```python
from build123d import *

# Parameters (mm, degrees)
SKETCH1_W           = 90
SKETCH1_H           = 60
SKETCH1_W_2         = 13.5
SKETCH1_H_2         = 54
SKETCH1_W_3         = 59.25
SKETCH1_H_3         = 43
BOSS_EXTRUDE3_DEPTH = 1.25
SKETCH1_6_W         = 100
SKETCH1_6_H         = 70
SKETCH1_6_R         = 1.5
SKETCH1_6_W_2       = 90
SKETCH1_6_H_2       = 60
BOSS_EXTRUDE4_DEPTH = 2.5


with BuildPart() as part:
    # Sketch1 → Boss-Extrude3 (new body)
    with BuildSketch(Plane.XY):
        with Locations((45, 30)):
            Rectangle(SKETCH1_W, SKETCH1_H)
        with Locations((81.5, 30.5)):
            Rectangle(SKETCH1_W_2, SKETCH1_H_2, mode=Mode.SUBTRACT)
        with Locations((38.125, 30)):
            Rectangle(SKETCH1_W_3, SKETCH1_H_3, mode=Mode.SUBTRACT)
    extrude(amount=-BOSS_EXTRUDE3_DEPTH)

    # Sketch1_6 → Boss-Extrude4 (add)
    with BuildSketch(Plane.XY):
        with Locations((45, 30)):
            Rectangle(SKETCH1_6_W, SKETCH1_6_H)
        with Locations((92.5, -2.5)):
            Circle(SKETCH1_6_R, mode=Mode.SUBTRACT)
        with Locations((92.5, 62.5)):
            Circle(SKETCH1_6_R, mode=Mode.SUBTRACT)
        with Locations((-2.5, 62.5)):
            Circle(SKETCH1_6_R, mode=Mode.SUBTRACT)
        with Locations((-2.5, -2.5)):
            Circle(SKETCH1_6_R, mode=Mode.SUBTRACT)
        with Locations((45, 30)):
            Rectangle(SKETCH1_6_W_2, SKETCH1_6_H_2, mode=Mode.SUBTRACT)
    extrude(amount=-BOSS_EXTRUDE4_DEPTH)


solid = part.part
```
Could you check a few things on this model? Use its own coordinates, in mm. A direction names the side the tool comes from. Coordinates: 2 decimals unless noted, no trailing zeros. Order: outer loops, then holes, each group sorted by start corner. A loop starts at its lowest first (then second) coordinate and runs counter-clockwise, first axis right, second up. Notation, with made-up numbers: M 78,-40 L 132,-40 A10 cw 132,-26 Z; hole C 77.5,5.25 d2. An arc over 180 degrees is marked long. Use a Markdown table: item, result. Add a question column.
Q1. Which directions (+Z, -Z, +X, -X, +Y, -Y) give clear straight access to the entire face, cutting with the end or side of a thin tool? Please do faces 4 (the flat face through (34, 4, -1.25)), 5 (the cylindrical face through (93.306, 63.765, -1.232)).
Q2. I want a section at D-D on y = 62.5. List the corners of the cut face in (x, z) for me, then the cut area to 3 significant figures.
Q3. I want a section at C-C on x = -2.5. List the corners of the cut face in (y, z) for me.
Q4. If I drill on L1, parallel to Y at x = 92.5, z = -1.55; L2, parallel to X at y = 40.5, z = -0.8; L3, parallel to X at y = 51, z = -1.8, over which ranges is the centre line in solid material (lowest first)?
Q5. I want a section at A-A on x = 84. List the corners of the cut face in (y, z) for me.
Q6. I want a section at B-B on y = 16. List the corners of the cut face in (x, z) for me.
Q7. We'd pull the mould along Y, two halves only. Please class faces 1 (the flat face through (44, 54, 0)), 2 (the flat face through (44, 65, -1)), 3 (the cylindrical face through (-2.695, 63.987, -1.232)): pulls with the +Y half, pulls with the -Y half, needs draft (parallel to the pull), parting line crosses it, or undercut.
Checked values:
| question | item | result |
|---|---|---|
| 1 | face 4 | -Z |
| 1 | face 5 | +Z, -Z |
| 2 | outline | M -5,-2.5 L -4,-2.5 L -4,0 L -5,0 Z; M -1,-2.5 L 91,-2.5 L 91,0 L -1,0 Z; M 94,-2.5 L 95,-2.5 L 95,0 L 94,0 Z |
| 2 | area | 235 mm² |
| 3 | outline | M -5,-2.5 L -4,-2.5 L -4,0 L -5,0 Z; M -1,-2.5 L 61,-2.5 L 61,0 L -1,0 Z; M 64,-2.5 L 65,-2.5 L 65,0 L 64,0 Z |
| 4 | L1 | -5 to -4, -1 to 61, 64 to 65 |
| 4 | L2 | -5 to 8.5, 67.75 to 74.75, 88.25 to 95 |
| 4 | L3 | -5 to 0, 90 to 95 |
| 5 | outline | M -5,-2.5 L 0,-2.5 L 0,-1.25 L 3.5,-1.25 L 3.5,0 L -5,0 Z; M 57.5,-1.25 L 60,-1.25 L 60,-2.5 L 65,-2.5 L 65,0 L 57.5,0 Z |
| 6 | outline | M -5,-2.5 L 0,-2.5 L 0,-1.25 L 8.5,-1.25 L 8.5,0 L -5,0 Z; M 67.75,-1.25 L 74.75,-1.25 L 74.75,0 L 67.75,0 Z; M 88.25,-1.25 L 90,-1.25 L 90,-2.5 L 95,-2.5 L 95,0 L 88.25,0 Z |
| 7 | face 1 | needs draft |
| 7 | face 2 | pulls with the +Y half |
| 7 | face 3 | undercut |
